Design review of the part built by this model. Coordinates are the model's own, in mm. Coordinates: 2 decimals unless noted, no trailing zeros. Answer in a Markdown table with one row per item.
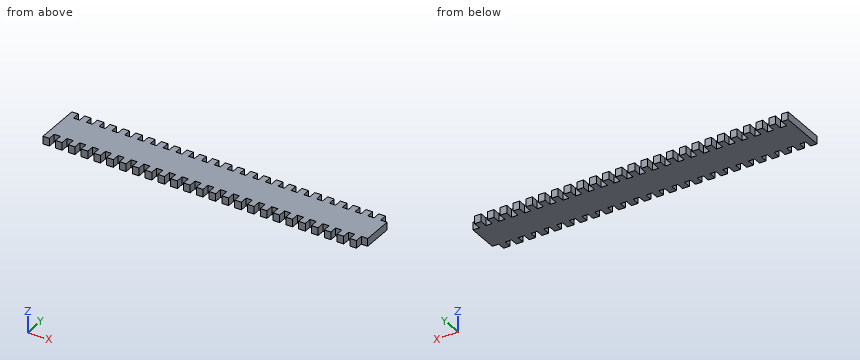
from build123d import *

# Parameters (mm, degrees)
BOSS_EXTRU_1_DEPTH      = 6
ESQUISSE2_W             = 0.2
ESQUISSE2_H             = 36
ENL_V_MAT_EXTRU_1_DEPTH = 10
ESQUISSE3_W             = 0.2
ESQUISSE3_H             = 24
BOSS_EXTRU_2_DEPTH      = 6


with BuildPart() as part:
    # Esquisse1 → Boss.-Extru.1 (new body)
    with BuildSketch(Plane.XY):
        Polygon((0, -18), (0, 18), (5.2, 18), (5.2, 12), (10, 12), (10, 18), (15.2, 18), (15.2, 12), (20, 12), (20, 18), (25.2, 18), (25.2, 12), (30, 12), (30, 18), (35.2, 18), (35.2, 12), (40, 12), (40, 18), (45.2, 18), (45.2, 12), (50, 12), (50, 18), (55.2, 18), (55.2, 12), (60, 12), (60, 18), (65.2, 18), (65.2, 12), (70, 12), (70, 18), (75.2, 18), (75.2, 12), (80, 12), (80, 18), (85.2, 18), (85.2, 12), (90, 12), (90, 18), (95.2, 18), (95.2, 12), (100, 12), (100, 18), (105.2, 18), (105.2, 12), (110, 12), (110, 18), (115.2, 18), (115.2, 12), (120, 12), (120, 18), (125.2, 18), (125.2, 12), (130, 12), (130, 18), (135.2, 18), (135.2, 12), (140, 12), (140, 18), (145.2, 18), (145.2, 12), (150, 12), (150, 18), (155.2, 18), (155.2, 12), (160, 12), (160, 18), (165.2, 18), (165.2, 12), (170, 12), (170, 18), (175.2, 18), (175.2, 12), (180, 12), (180, 18), (185.2, 18), (185.2, 12), (190, 12), (190, 18), (195.2, 18), (195.2, 12), (200, 12), (200, 18), (205.2, 18), (205.2, 12), (210, 12), (210, 18), (215.2, 18), (215.2, 12), (220, 12), (220, 18), (225.2, 18), (225.2, 12), (230, 12), (230, 18), (235.2, 18), (235.2, 12), (240, 12), (240, 18), (245.2, 18), (245.2, 12), (250, 12), (250, -12), (245.2, -12), (245.2, -18), (240, -18), (240, -12), (235.2, -12), (235.2, -18), (230, -18), (230, -12), (225.2, -12), (225.2, -18), (220, -18), (220, -12), (215.2, -12), (215.2, -18), (210, -18), (210, -12), (205.2, -12), (205.2, -18), (200, -18), (200, -12), (195.2, -12), (195.2, -18), (190, -18), (190, -12), (185.2, -12), (185.2, -18), (180, -18), (180, -12), (175.2, -12), (175.2, -18), (170, -18), (170, -12), (165.2, -12), (165.2, -18), (160, -18), (160, -12), (155.2, -12), (155.2, -18), (150, -18), (150, -12), (145.2, -12), (145.2, -18), (140, -18), (140, -12), (135.2, -12), (135.2, -18), (130, -18), (130, -12), (125.2, -12), (125.2, -18), (120, -18), (120, -12), (115.2, -12), (115.2, -18), (110, -18), (110, -12), (105.2, -12), (105.2, -18), (100, -18), (100, -12), (95.2, -12), (95.2, -18), (90, -18), (90, -12), (85.2, -12), (85.2, -18), (80, -18), (80, -12), (75.2, -12), (75.2, -18), (70, -18), (70, -12), (65.2, -12), (65.2, -18), (60, -18), (60, -12), (55.2, -12), (55.2, -18), (50, -18), (50, -12), (45.2, -12), (45.2, -18), (40, -18), (40, -12), (35.2, -12), (35.2, -18), (30, -18), (30, -12), (25.2, -12), (25.2, -18), (20, -18), (20, -12), (15.2, -12), (15.2, -18), (10, -18), (10, -12), (5.2, -12), (5.2, -18), align=None)
    extrude(amount=BOSS_EXTRU_1_DEPTH)

    # Esquisse2 → Enlèv. mat.-Extru.1 (cut)
    with BuildSketch(Plane.XY.offset(6)):
        with Locations((0.1, 0)):
            Rectangle(ESQUISSE2_W, ESQUISSE2_H)
    extrude(amount=-ENL_V_MAT_EXTRU_1_DEPTH, mode=Mode.SUBTRACT)

    # Esquisse3 → Boss.-Extru.2 (add)
    with BuildSketch(Plane.XY.offset(6)):
        with Locations((250.1, 0)):
            Rectangle(ESQUISSE3_W, ESQUISSE3_H)
    extrude(amount=-BOSS_EXTRU_2_DEPTH)


solid = part.part
(1) Add section A-A, the plane y = 14.5. Give the number of separate pieces and of enclosed holes in the cut face, and give its area (3 significant figures).
Return value:
| item | result |
|---|---|
| separate pieces | 25 |
| enclosed holes | 0 |
| area | 779 mm2 |
(2) For line 1 along Y through (x, z) = (35.5, 2.55), list the stretches that pass through material, from the lowest coordinate up. Write a range as from..to.
Return value:
| item | result |
|---|---|
| line 1 | y = -12..12 |
(3) Insertion check: pin 1 Ø2.5 at (x, z) = (37, 3) entering from +Y; pin 2 Ø1.8 at (y, z) = (-15.5, 4) entering from +X; pin 3 Ø2.5 at (x, z) = (67, 2) entering from -Y. Each pin has a flat end and moves straight along its axis. Give the tip position at first contact, or say it passes through.
Return value:
| item | result |
|---|---|
| pin 1 | stops at y = 12 |
| pin 2 | stops at x = 245.2 |
| pin 3 | stops at y = -12 |
